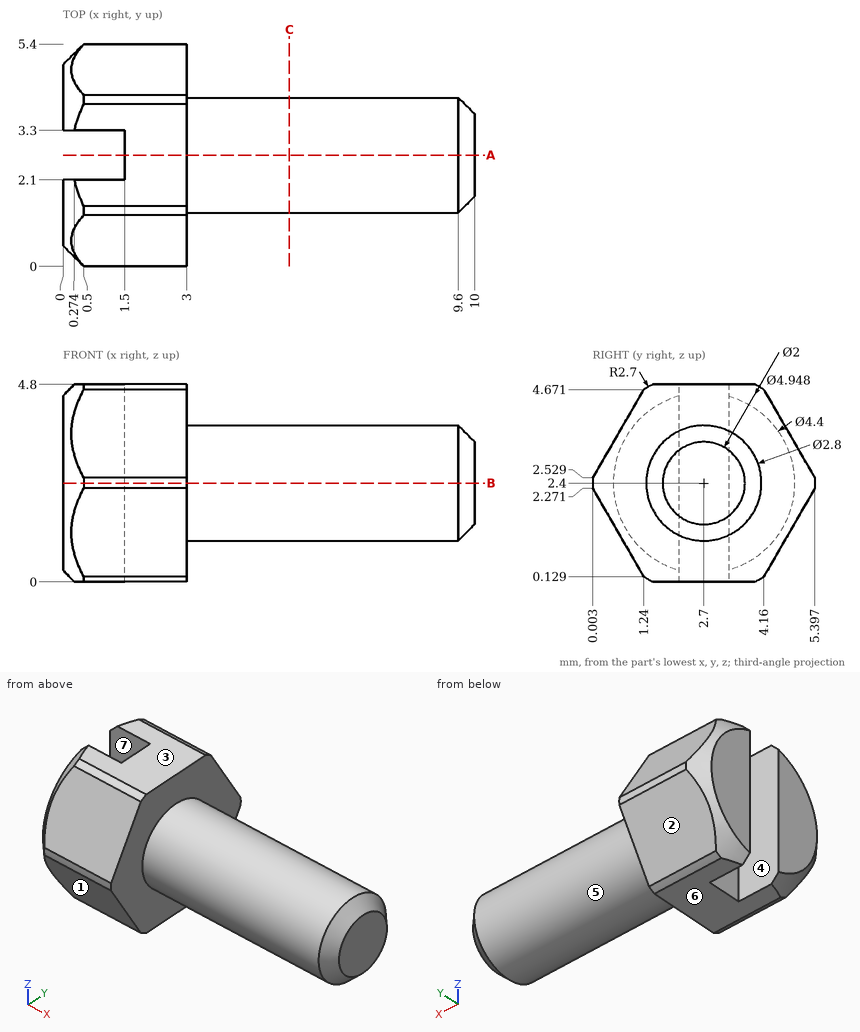
Geometry: see drawing. Coordinates: mm, zero at the bounding-box minimum. A direction names the side the tool comes from. Give positions to 0.01 mm unless a question says otherwise; leave off trailing zeros. Loops run counter-clockwise (first coordinate to the right, second up) from the corner with the lowest first, then second, coordinate; pieces in that order, holes last. Notation, with made-up numbers: (3, 68.5) - (18, 68.5) arc R33 cw to (18, 104.5) - close; hole circle Ø2 at (55, -32.75). An arc over 180 degrees is marked (long way). Answer as CSV lines item,"result". Start each with the question number.
1. Section B-B, the plane z = 2.4. Return loops of the section in (x, y), plus the area to 3 significant figures.
2. Draft query along Y for the marked faces 1, 2, 3 and 4. Return one class per face: released by +Y, released by -Y, zero draft, split by the parting line, or undercut.
3. Pin query (flat end, axial travel): P1, Ø2, axis at x = 1, z = 4, coming from the +Y side (1 decimal); P2, Ø0.8, axis at x = 1, z = 1.5, coming from the +Y side. Return the tip coordinate at first contact, or that it passes through.
4. Section C-C, the plane x = 5.5. Return loops of the section in (y, z).
5. Ray query, L1, parallel to X at y = 3.2, z = 0.95; L2, parallel to X at y = 1.5, z = 1.55; L3, parallel to Y at x = 2, z = 4.4. Return the intervals inside material, ascending.
6. Section A-A, the plane y = 2.7. Return loops of the section in (x, z).
7. Reachability of the marked faces 5, 6 and 7 from +Z, -Z, +X, -X, +Y, -Y: full face, straight path, thin tool, end or side. Return the list, or none.
Answers:
1,outline,"(0, 0.5) - (0.5, 0) - (3, 0) - (3, 1.3) - (9.6, 1.3) - (10, 1.7) - (10, 3.7) - (9.6, 4.1) - (3, 4.1) - (3, 5.4) - (0.5, 5.4) - (0, 4.9) - (0, 3.3) - (1.5, 3.3) - (1.5, 2.1) - (0, 2.1) - close"
1,area,"33.6 mm2"
2,face 1,"released by -Y"
2,face 2,"released by +Y"
2,face 3,"zero draft"
2,face 4,"undercut"
3,P1,"stops at y = 5.1"
3,P2,"stops at y = 5.18"
4,outline,"circle Ø2.8 at (2.7, 2.4)"
5,L1,"x = 1.5 to 3"
5,L2,"x = 0 to 3"
5,L3,"y = 1.08 to 4.32"
6,outline,"(1.5, 0) - (3, 0) - (3, 1) - (9.6, 1) - (10, 1.4) - (10, 3.4) - (9.6, 3.8) - (3, 3.8) - (3, 4.8) - (1.5, 4.8) - close"
7,face 5,"+X"
7,face 6,"-Z, +X, -X, +Y, -Y"
7,face 7,"+Z, -Z, -X"
